```python
from build123d import *

# Parameters (mm, degrees)
SKETCH_1_W      = 99.8
SKETCH_1_H      = 44.8
EXTRUDE_1_DEPTH = 4


# Read off the part's stored shape, not the designer's step: M5 扁圆形螺钉的柱孔
with BuildPart() as part:
    # 草图1 → 凸台-拉伸1 (new body)
    with BuildSketch(Plane(origin=(0, 0, 0), x_dir=(1, 0, 0), z_dir=(0, 1, 0))):
        Rectangle(SKETCH_1_W, SKETCH_1_H)
    extrude(amount=EXTRUDE_1_DEPTH)

    # M5 扁圆形螺钉的柱孔 outline → M5 扁圆形螺钉的柱孔 (revolve, cut)
    with BuildSketch(Plane(origin=(43.9, 0, -15.4), x_dir=(1, 0, 0), z_dir=(0, 0, 1))):
        Polygon((2.75, 3.3), (2.75, 4), (0, 4), (0, 0), (5.025, 0), (5, 0.025), (5, 3.3), align=None)
    revolve(axis=Axis((43.9, 0, -15.4), (0, 1, 0)), mode=Mode.SUBTRACT)

    # Hole Wizard M5 2 outline → Hole Wizard M5 2 (revolve, cut)
    with BuildSketch(Plane(origin=(43.9, 0, 15.4), x_dir=(1, 0, 0), z_dir=(0, 0, 1))):
        Polygon((0, 0), (5.025, 0), (5, 0.025), (5, 3.3), (2.75, 3.3), (2.75, 4), (0, 4), align=None)
    revolve(axis=Axis((43.9, 0, 15.4), (0, 1, 0)), mode=Mode.SUBTRACT)

    # Hole Wizard M5 3 outline → Hole Wizard M5 3 (revolve, cut)
    with BuildSketch(Plane(origin=(-43.9, 0, 15.4), x_dir=(1, 0, 0), z_dir=(0, 0, 1))):
        Polygon((0, 0), (5.025, 0), (5, 0.025), (5, 3.3), (2.75, 3.3), (2.75, 4), (0, 4), align=None)
    revolve(axis=Axis((-43.9, 0, 15.4), (0, 1, 0)), mode=Mode.SUBTRACT)

    # Hole Wizard M5 4 outline → Hole Wizard M5 4 (revolve, cut)
    with BuildSketch(Plane(origin=(-43.9, 0, -15.4), x_dir=(1, 0, 0), z_dir=(0, 0, 1))):
        Polygon((0, 0), (5.025, 0), (5, 0.025), (5, 3.3), (2.75, 3.3), (2.75, 4), (0, 4), align=None)
    revolve(axis=Axis((-43.9, 0, -15.4), (0, 1, 0)), mode=Mode.SUBTRACT)


solid = part.part
```
Check sheet for the modelled part. Datum: model origin and axes. Units: mm. A direction names the side the tool comes from. Round coordinates to 2 decimals unless told otherwise and drop trailing zeros. Order: outer loops, then holes, each group sorted by start corner. A loop starts at its lowest first (then second) coordinate and runs counter-clockwise, first axis right, second up. Notation, with made-up numbers: (-27.5, -1) -> (17.5, -1) arc R18 ccw to (17.5, 14) -> close; hole circle Ø5 at (3, 32). An arc over 180 degrees is marked (long way). Use CSV: the item, a comma, the result in double quotes.
(1) Cross-section at C-C (y = 1.9). Record the boundary of the cut face in (x, z), and give its area (3 significant figures).
Worked out:
outline,"(-49.9, -22.4) -> (49.9, -22.4) -> (49.9, 22.4) -> (-49.9, 22.4) -> close; hole circle Ø10 at (-43.9, -15.4); hole circle Ø10 at (-43.9, 15.4); hole circle Ø10 at (43.9, -15.4); hole circle Ø10 at (43.9, 15.4)"
area,"4,160 mm²"
(2) Cross-section at B-B (z = -15.4). Record the boundary of the cut face in (x, y) (3 decimals), and give its area (3 significant figures).
Worked out:
outline,"(-49.9, 0) -> (-48.925, 0) -> (-48.9, 0.025) -> (-48.9, 3.3) -> (-46.65, 3.3) -> (-46.65, 4) -> (-49.9, 4) -> close; (-41.15, 3.3) -> (-38.9, 3.3) -> (-38.9, 0.025) -> (-38.875, 0) -> (38.875, 0) -> (38.9, 0.025) -> (38.9, 3.3) -> (41.15, 3.3) -> (41.15, 4) -> (-41.15, 4) -> close; (46.65, 3.3) -> (48.9, 3.3) -> (48.9, 0.025) -> (48.925, 0) -> (49.9, 0) -> (49.9, 4) -> (46.65, 4) -> close"
area,"325 mm²"
(3) Depth check by flat-ended pin: pin 1 (6 mm diameter, centred on x = -43.9, z = -15.4, fed in from -Y). Enter the tip coordinate at first touch or a pass-through.
Worked out:
pin 1,"y = 3.3"
(4) Tool access check on faces 4 (the face through (46, 3.3, -13)), 5 (the face through (-1, 0, 0)). Record the directions out of +Z, -Z, +X, -X, +Y, -Y that give a thin tool (end or side, any length) a straight path to the whole face; none if there is none.
Worked out:
face 4,"-Y"
face 5,"+Z, -Z, +X, -X, -Y"
(5) Material ranges on line 1 along X through (y, z) = (3.7, -15.4); line 2 along X through (y, z) = (2.15, 15.4); line 3 along Z through (x, y) = (-43.9, 3.7), recorded low to high. Write a range as from..to.
Worked out:
line 1,"-49.9..-46.65, -41.15..41.15, 46.65..49.9"
line 2,"-49.9..-48.9, -38.9..38.9, 48.9..49.9"
line 3,"-22.4..-18.15, -12.65..12.65, 18.15..22.4"
(6) Draft check along Z on faces 1 (the face through (-1, 2, -22.4)), 2 (the face through (46, 3.3, 18)), 3 (the face through (49.9, 2, 0)). Enter one of: pulls with the +Z half, pulls with the -Z half, needs draft (parallel to the pull), parting line crosses it, or undercut.
Worked out:
face 1,"pulls with the -Z half"
face 2,"undercut"
face 3,"needs draft"
(7) Cross-section at A-A (x = 43.9). Record the boundary of the cut face in (y, z) (3 decimals), and give its area (3 significant figures).
Worked out:
outline,"(0, -22.4) -> (4, -22.4) -> (4, -18.15) -> (3.3, -18.15) -> (3.3, -20.4) -> (0.025, -20.4) -> (0, -20.425) -> close; (0, -10.375) -> (0.025, -10.4) -> (3.3, -10.4) -> (3.3, -12.65) -> (4, -12.65) -> (4, 12.65) -> (3.3, 12.65) -> (3.3, 10.4) -> (0.025, 10.4) -> (0, 10.375) -> close; (0, 20.425) -> (0.025, 20.4) -> (3.3, 20.4) -> (3.3, 18.15) -> (4, 18.15) -> (4, 22.4) -> (0, 22.4) -> close"
area,"105 mm²"
